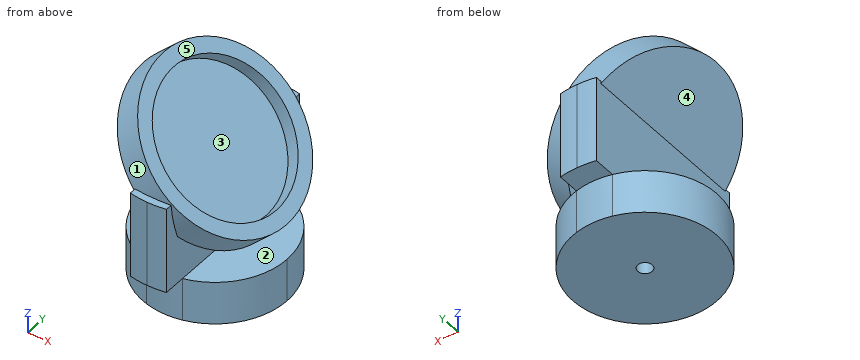
```python
from build123d import *

# Parameters (mm, degrees)
F3_R     = 12
F3_R_2   = 10
F4_DEPTH = 2
F5_DEPTH = 12
F6_R     = 1
F7_DEPTH = 6
F8_DEPTH = 2


with BuildPart() as f4:
    # F3 (on 3pt) → F4 (new body, symmetric)
    with BuildSketch(Plane(origin=(0, 0, 0), x_dir=(0.7071067812, 0, -0.7071067812), z_dir=(-0.7071067812, 0, -0.7071067812))):
        Circle(F3_R)
        Circle(F3_R_2, mode=Mode.SUBTRACT)
        Circle(F3_R_2)
    extrude(amount=F4_DEPTH, both=True)

    # F0 (on Top) → F5 (join)
    with BuildSketch(Plane.XY):
        with BuildLine():
            ThreePointArc((-2.5, -12.7573508222), (-1.2558740605, -12.9391955061), (0, -13))
            Line((0, -13), (0, 0))
            Line((0, 0), (-2.5, 0))
            Line((-2.5, 0), (-2.5, -12.7573508222))
        make_face()
        with BuildLine():
            Line((0, 0), (0, 13))
            ThreePointArc((0, 13), (-1.2558740605, 12.9391955061), (-2.5, 12.7573508222))
            Line((-2.5, 12.7573508222), (-2.5, 0))
            Line((-2.5, 0), (0, 0))
        make_face()
        with BuildLine():
            Line((2.5, 0), (2.5, 12.7573508222))
            ThreePointArc((2.5, 12.7573508222), (1.2558740605, 12.9391955061), (0, 13))
            Line((0, 13), (0, 0))
            Line((0, 0), (2.5, 0))
        make_face()
        with BuildLine():
            ThreePointArc((0, -13), (1.2558740605, -12.9391955061), (2.5, -12.7573508222))
            Line((2.5, -12.7573508222), (2.5, 0))
            Line((2.5, 0), (0, 0))
            Line((0, 0), (0, -13))
        make_face()
    extrude(amount=-F5_DEPTH)

    # F6 (on face) → F7 (join)
    with BuildSketch(Plane(origin=(0, 0, -12), x_dir=(1, 0, 0), z_dir=(0, 0, -1))):
        with BuildLine():
            ThreePointArc((2.5, -9.6824583655), (7.9056941504, -6.123724357), (10, 0))
            ThreePointArc((10, 0), (7.9056941504, 6.123724357), (2.5, 9.6824583655))
            Line((2.5, 9.6824583655), (2.5, -9.6824583655))
        make_face()
        with BuildLine():
            Line((-2.5, -9.6824583655), (-2.5, 9.6824583655))
            ThreePointArc((-2.5, 9.6824583655), (-10, 0), (-2.5, -9.6824583655))
        make_face()
        with BuildLine():
            Line((2.5, -9.6824583655), (2.5, 9.6824583655))
            ThreePointArc((2.5, 9.6824583655), (0, 10), (-2.5, 9.6824583655))
            Line((-2.5, 9.6824583655), (-2.5, -9.6824583655))
            ThreePointArc((-2.5, -9.6824583655), (0, -10), (2.5, -9.6824583655))
        make_face()
        Circle(F6_R, mode=Mode.SUBTRACT)
    extrude(amount=F7_DEPTH)

    # F3 (on 3pt) → F8 (cut)
    with BuildSketch(Plane(origin=(0, 0, 0), x_dir=(0.7071067812, 0, -0.7071067812), z_dir=(-0.7071067812, 0, -0.7071067812))):
        Circle(F3_R_2)
    extrude(amount=-F8_DEPTH, mode=Mode.SUBTRACT)


solid = f4.part
```
The model under review builds one solid part; all positions refer to its coordinate system, in mm. Face numbers are marked on the shaded views. A direction names the side the tool comes from. Round coordinates to 2 decimals unless told otherwise and drop trailing zeros. Write each loop counter-clockwise with the first axis right and the second up, starting at its lowest first coordinate (ties: lowest second). Pieces come first, ordered by that corner, then holes.
(1) Mouldability with a two-part tool opening along Y and no side actions: class the marked faces 1, 2 and 3 as +Y half, -Y half, draft (parallel to the pull), parting line (faces both ways), or undercut.
(2) Insertion check: pin 1 (1 mm diameter, centred on x = 0, y = -11.5, fed in from -Z); pin 2 (2.5 mm diameter, centred on x = 0, y = 0, fed in from +Z); pin 3 (0.6 mm diameter, centred on x = 0, y = 12, fed in from +Z). Each pin has a flat end and moves straight along its axis. Give the tip position at first contact, or say it passes through.
(3) We need section A-A on z = -11. Give the boundary of the cut face in (x, y), and give its area (3 significant figures).
(4) We need section B-B on y = 6.75. Give the boundary of the cut face in (x, z).
(5) We need section C-C on y = -8. Give the boundary of the cut face in (x, z), and give its area (3 significant figures).
(6) We need section D-D on y = -11.25. Give the boundary of the cut face in (x, z), and give its area (3 significant figures).
(7) Wall thickness on L1, parallel to Y at x = 0, z = -16.65; L2, parallel to X at y = 1, z = -5.75; L3, parallel to X at y = -5, z = -6.75: over which ranges is each line inside the solid? List them lowest first.
(8) Machinability: for the marked faces 4 and 5, which of the approach directions +Z, -Z, +X, -X, +Y, -Y give a long, thin tool a straight path to every point of the face, cutting with its end or side? Answer none if there is none.
Findings below:
1. face 1: parting line
1. face 2: draft
1. face 3: undercut
2. pin 1: stops at z = -12
2. pin 2: stops at z = 1.25
2. pin 3: stops at z = 3.03
3. outline: (-2.5, -12.76) arc R13 ccw to (2.5, -12.76) - (2.5, 12.76) arc R13 ccw to (-2.5, 12.76) - close
3. area: 129 mm2
4. outline: (-8.43, 5.6) - (-2.5, -0.33) - (-2.5, -12) - (-7.38, -12) - (-7.38, -18) - (7.38, -18) - (7.38, -12) - (2.5, -12) - (2.5, -5.33) - (5.6, -8.43) - (8.43, -5.6) - (6.63, -3.8) - (5.22, -5.22) - (-5.22, 5.22) - (-3.8, 6.63) - (-5.6, 8.43) - close
5. outline: (-7.74, 4.91) - (-2.5, -0.33) - (-2.5, -12) - (-6, -12) - (-6, -18) - (6, -18) - (6, -12) - (2.5, -12) - (2.5, -5.33) - (4.91, -7.74) - (7.74, -4.91) - (5.66, -2.83) - (4.24, -4.24) - (-4.24, 4.24) - (-2.83, 5.66) - (-4.91, 7.74) - close
5. area: 165 mm2
6. outline: (-4.37, 1.54) - (-2.5, -0.33) - (-2.5, -12) - (2.5, -12) - (2.5, -3.41) - (4.37, -1.54) - (-1.54, 4.37) - close
6. area: 80.2 mm2
7. L1: y = -10 to -1, 1 to 10
7. L2: x = -2.5 to 2.5, 2.92 to 5.75, 8.32 to 8.58
7. L3: x = -2.5 to 2.5, 3.92 to 8.68
8. face 4: -X, +Y, -Y
8. face 5: +Z, +X, +Y, -Y
